```python
from build123d import *

# Parameters (mm, degrees)
SKETCH003_W             = 16
SKETCH003_H             = 16
PAD_DEPTH               = 10
PAD001_DEPTH            = 5
CHAMFER_SIZE            = 2
SKETCH002_R             = 15
SKETCH002_R_2           = 8
POCKET_DEPTH            = 30.001
SKETCH007_R             = 1
POCKET002_DEPTH         = 4
BODY001_PLACEMENT_ANGLE = 180


with BuildPart() as part:
    # Sketch003 → Pad (new body)
    with BuildSketch(Plane.XY):
        Rectangle(SKETCH003_W, SKETCH003_H)
    extrude(amount=PAD_DEPTH)

    # Sketch001 → Pad001 (join)
    with BuildSketch(Plane.XZ):
        with BuildLine():
            Line((8, 10), (8, 22))
            ThreePointArc((8, 22), (0, 30), (-8, 22))
            Line((-8, 22), (-8, 10))
            Line((-8, 10), (8, 10))
        make_face()
        with BuildLine():
            ThreePointArc((-2.4377, 25.481396), (0, 17.75), (2.4377, 25.481396))
            Line((1.34002, 26.25), (2.4377, 25.481396))
            Line((-1.34002, 26.25), (1.34002, 26.25))
            Line((-1.34002, 26.25), (-2.4377, 25.481396))
        make_face(mode=Mode.SUBTRACT)
    extrude(amount=PAD001_DEPTH)

    # Chamfer
    chamfer_edges = [part.edges().sort_by_distance(p)[0] for p in [
        (0, -5, 10),
        (0, 0, 10),
    ]]
    chamfer(chamfer_edges, length=CHAMFER_SIZE)

    # Sketch002 → Pocket (cut, through all)
    with BuildSketch(Plane.XY):
        Circle(SKETCH002_R)
        Circle(SKETCH002_R_2, mode=Mode.SUBTRACT)
    extrude(amount=POCKET_DEPTH, mode=Mode.SUBTRACT)

    # Sketch007 (on Face13 of Pocket) → Pocket002 (cut)
    with BuildSketch(Plane(origin=(0, 0, 0), x_dir=(1, 0, 0), z_dir=(0, 0, -1))):
        Circle(SKETCH007_R)
    extrude(amount=-POCKET002_DEPTH, mode=Mode.SUBTRACT)


with BuildPart() as part_1:
    # Body001 placement: moved
    add(part.part.moved(Location((0, 0, 44.2))).rotate(Axis((0, 0, 44.2), (1, 0, 0)), BODY001_PLACEMENT_ANGLE))


solid = part_1.part
```
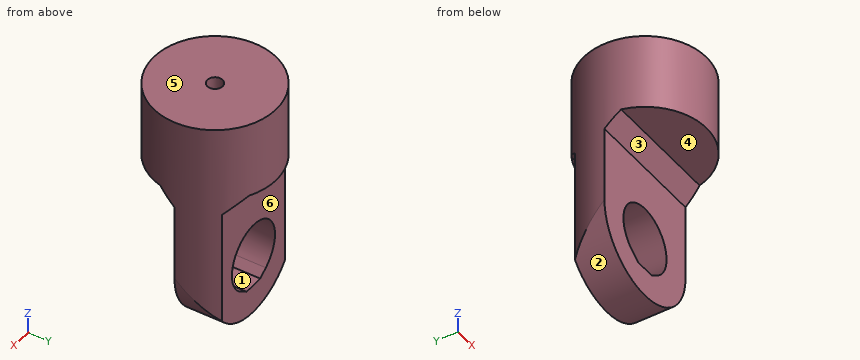
Read the model definition and answer for the solid it produces. Units are mm, in the model's axes. Face numbers are marked on the shaded views. A direction names the side the tool comes from. Coordinates: 2 decimals unless noted, no trailing zeros. Loops run counter-clockwise (first coordinate to the right, second up) from the corner with the lowest first, then second, coordinate; pieces in that order, holes last. Notation, with made-up numbers: (23, 8) - (33, 8) arc R12 cw to (33, 28) - close; hole circle Ø3 at (9.5, 10.25). An arc over 180 degrees is marked (long way). Answer in a Markdown table with one row per item.
1. Given pin 1 (0.5 mm diameter, centred on x = -1.5, y = 7.5, fed in from -Z); pin 2 (1 mm diameter, centred on x = -3, z = 31, fed in from -Y); pin 3 (1 mm diameter, centred on y = -2, z = 31, fed in from -X); pin 4 (2 mm diameter, centred on y = 1, z = 18.5, fed in from -X), each flat-ended and moving along its own axis, determine where each tip first touches the part or whether it passes through.
Conclusion:
| item | result |
|---|---|
| pin 1 | stops at z = 34.2 |
| pin 2 | stops at y = 0 |
| pin 3 | passes through |
| pin 4 | stops at x = -7.53 |
2. Which of the six approach directions +Z, -Z, +X, -X, +Y, -Y give full straight-line access (tool end or side, diameter ignored) to the marked faces 4, 5 and 6?
Conclusion:
| item | result |
|---|---|
| face 4 | -Z, +X, -X, -Y |
| face 5 | +Z, +X, -X, +Y, -Y |
| face 6 | -Z, +X, -X, +Y |
3. Find section D-D, the plane x = -3. Write down the section's boundary in (y, z).
Conclusion:
| item | result |
|---|---|
| outline | (-7.42, 34.2) - (-2, 34.2) - (0, 32.2) - (0, 25.21) - (5, 25.21) - (5, 32.2) - (7, 34.2) - (7.42, 34.2) - (7.42, 44.2) - (-7.42, 44.2) - close; (0, 14.78) - (5, 14.78) - (5, 19.19) - (0, 19.19) - close |
4. Straight lines are drawn through the part: line 1 (Z direction, x = 0, y = 1.95); line 2 (Y direction, x = -5, z = 16.75); line 3 (Y direction, x = 0, z = 41.5). For each, find the intervals that lie inside material, in ascending order.
Conclusion:
| item | result |
|---|---|
| line 1 | z = 14.2 to 17.95, 26.45 to 44.2 |
| line 2 | y = 0 to 5 |
| line 3 | y = -8 to -1, 1 to 8 |
5. Find section C-C, the plane y = 2.75. Write down the section's boundary in (x, z), then the cut area to 3 significant figures.
Conclusion:
| item | result |
|---|---|
| outline | (-7.51, 19.45) arc R8 ccw to (7.51, 19.45) - (7.51, 44.2) - (-7.51, 44.2) - close; hole (-2.44, 18.72) - (-1.34, 17.95) - (1.34, 17.95) - (2.44, 18.72) arc R4.25 ccw (long way) to start |
| area | 372 mm² |
6. Find section A-A, the plane z = 24. Write down the section's boundary in (x, y) (3 decimals), then the cut area to 3 significant figures.
Conclusion:
| item | result |
|---|---|
| outline | (-8, 0) - (-3.85, 0) - (-3.85, 5) - (-6.245, 5) arc R8 ccw to start; (3.85, 0) - (8, 0) arc R8 ccw to (6.245, 5) - (3.85, 5) - close |
| area | 35.9 mm² |
7. Determine the mould class of the marked faces 1, 2 and 3 for opening direction X: +X half, -X half, draft (parallel to the pull), parting line (faces both ways), or undercut.
Conclusion:
| item | result |
|---|---|
| face 1 | undercut |
| face 2 | parting line |
| face 3 | draft |
8. Find section B-B, the plane x = 0. Write down the section's boundary in (y, z), then the cut area to 4 significant figures.
Conclusion:
| item | result |
|---|---|
| outline | (-8, 34.2) - (-2, 34.2) - (0, 32.2) - (0, 26.45) - (5, 26.45) - (5, 32.2) - (7, 34.2) - (8, 34.2) - (8, 44.2) - (1, 44.2) - (1, 40.2) - (-1, 40.2) - (-1, 44.2) - (-8, 44.2) - close; (0, 14.2) - (5, 14.2) - (5, 17.95) - (0, 17.95) - close |
| area | 213.5 mm² |
